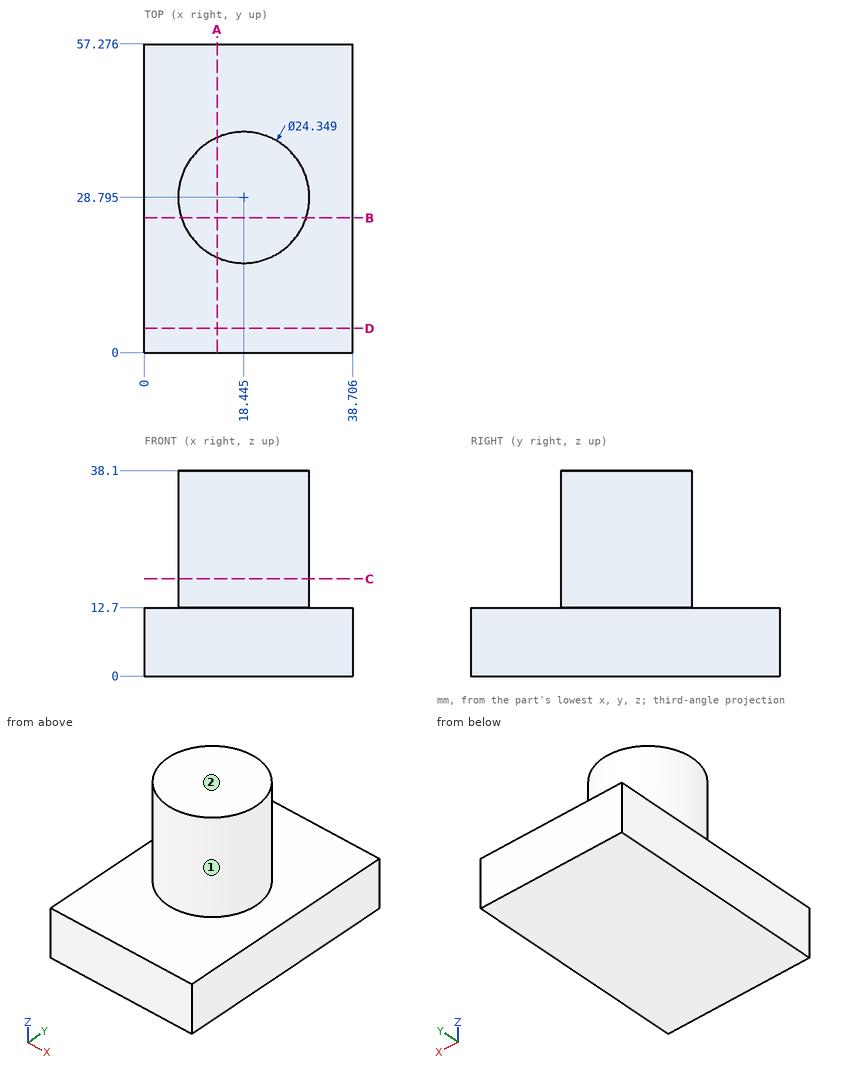
Can you work these out from the drawing? Everything is in mm from the part's minimum corner. A direction names the side the tool comes from. Round coordinates to 2 decimals unless told otherwise and drop trailing zeros. Write each loop counter-clockwise with the first axis right and the second up, starting at its lowest first coordinate (ties: lowest second). Pieces come first, ordered by that corner, then holes.
1. For the marked faces 1 and 2, which set-ups out of +Z, -Z, +X, -X, +Y, -Y let a thin tool reach every point of the face, with its end or its side?
2. I need wall thicknesses on L1, parallel to Z at x = 7, y = 20; L2, parallel to X at y = 17.5, z = 36 (1 decimal); L3, parallel to X at y = 33, z = 32.5. Which ranges of each line are inside material? Lowest first, please.
3. Suppose I cut it at D-D (y = 4.5). List the corners of the cut face in (x, z) for me.
4. Suppose I cut it at B-B (y = 25). List the corners of the cut face in (x, z) for me.
5. Suppose I cut it at C-C (z = 18). List the corners of the cut face in (x, y) for me (1 decimal), and give its area (3 significant figures).
6. Will these pins go through, and if not, where does the flat tip stop? pin 1 Ø3 at (x, y) = (29.5, 37.5) entering from -Z; pin 2 Ø4 at (x, y) = (32.5, 20) entering from +Z.
7. Suppose I cut it at A-A (x = 13.5). List the corners of the cut face in (y, z) for me.
Answer sheet:
1. face 1: +Z
1. face 2: +Z, +X, -X, +Y, -Y
2. L1: z = 0 to 12.7
2. L2: x = 13.9 to 23
2. L3: x = 7.02 to 29.87
3. outline: (0, 0) - (38.71, 0) - (38.71, 12.7) - (0, 12.7) - close
4. outline: (0, 0) - (38.71, 0) - (38.71, 12.7) - (30.01, 12.7) - (30.01, 38.1) - (6.88, 38.1) - (6.88, 12.7) - (0, 12.7) - close
5. outline: circle Ø24.3 at (18.4, 28.8)
5. area: 466 mm2
6. pin 1: stops at z = 0
6. pin 2: stops at z = 12.7
7. outline: (0, 0) - (57.28, 0) - (57.28, 12.7) - (39.92, 12.7) - (39.92, 38.1) - (17.67, 38.1) - (17.67, 12.7) - (0, 12.7) - close
